Study the drawing (mm; zero at the part's minimum x, y, z) and answer. Give positions to 0.01 mm unless a question says otherwise; leave off trailing zeros. Loops run counter-clockwise (first coordinate to the right, second up) from the corner with the lowest first, then second, coordinate; pieces in that order, holes last. Notation, with made-up numbers: M 66.25,60 L 120.25,60 A19 ccw 120.25,90 Z; hole C 60.5,81 d9. An arc over 180 degrees is marked long. Return JSON: item names as keys, results as strings.
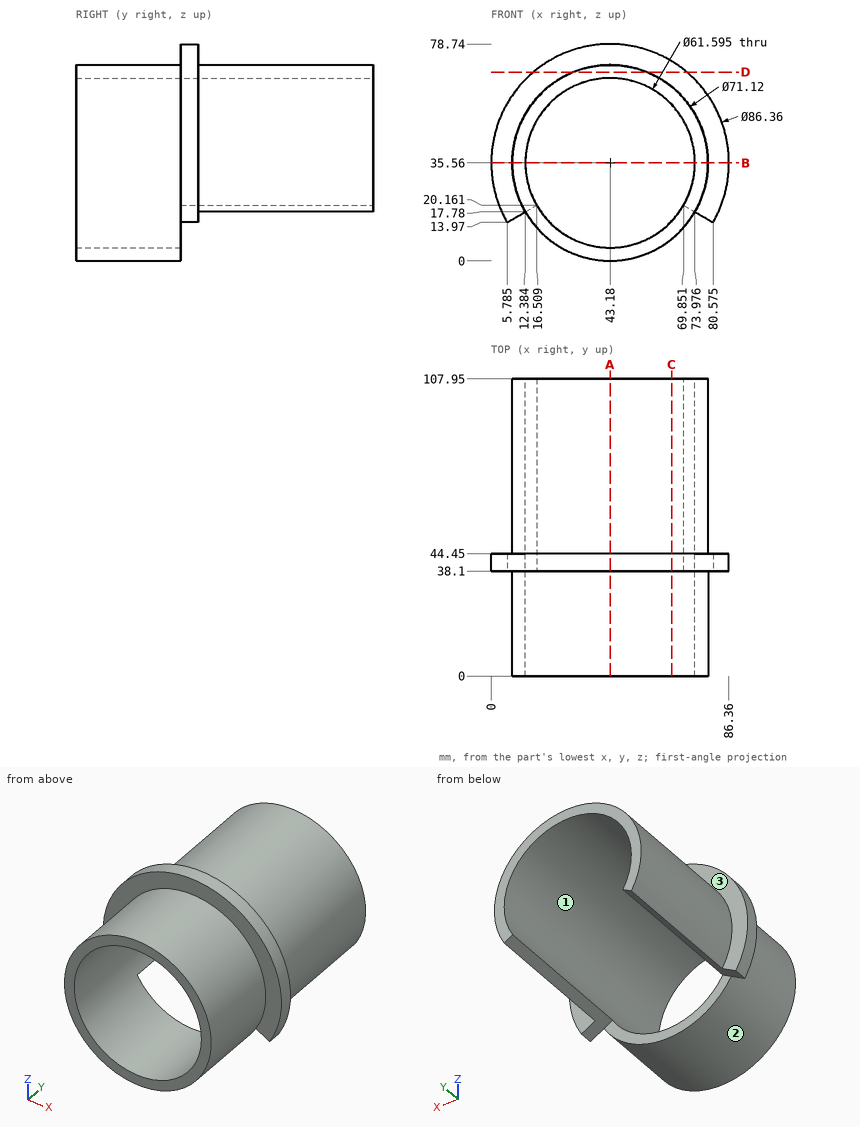
(1) Given pin 1 (1.5 mm diameter, centred on y = 46.5, z = 58.5, fed in from -X); pin 2 (1.5 mm diameter, centred on y = 33.5, z = 28.5, fed in from +X); pin 3 (5 mm diameter, centred on x = 12.5, z = 39, fed in from -Y); pin 4 (4 mm diameter, centred on y = 81.5, z = 47, fed in from -X), each flat-ended and moving along its own axis, determine where each tip first touches the part or whether it passes through.
Values follow:
{"pin 1": "x = 15.39", "pin 2": "x = 78.18", "pin 3": "y = 0", "pin 4": "x = 8.9"}
(2) The part is cut by section A-A (x = 43.18). Determine the outline of the cut face in (y, z).
Values follow:
{"outline": "M 0,0 L 38.1,0 L 38.1,4.76 L 0,4.76 Z; M 0,66.36 L 107.95,66.36 L 107.95,71.12 L 44.45,71.12 L 44.45,78.74 L 38.1,78.74 L 38.1,71.12 L 0,71.12 Z"}
(3) The part is cut by section D-D (z = 68.5). Determine the outline of the cut face in (x, y), and give its area (3 significant figures).
Values follow:
{"outline": "M 15.26,38.1 L 29.78,38.1 L 29.78,0 L 56.58,0 L 56.58,38.1 L 71.1,38.1 L 71.1,44.45 L 56.58,44.45 L 56.58,107.95 L 29.78,107.95 L 29.78,44.45 L 15.26,44.45 Z", "area": "3,080 mm²"}
(4) Straight lines are drawn through the part: line 1 along X through (y, z) = (82.5, 35.56); line 2 along Z through (x, y) = (43.18, 24.5); line 3 along Y through (x, z) = (78, 61). For each, find the intervals that lie inside material, in ascending order.
Values follow:
{"line 1": "7.62 to 12.38, 73.98 to 78.74", "line 2": "0 to 4.76, 66.36 to 71.12", "line 3": "38.1 to 44.45"}
(5) The part is cut by section B-B (z = 35.56). Determine the outline of the cut face in (x, y).
Values follow:
{"outline": "M 0,38.1 L 7.62,38.1 L 7.62,0 L 12.38,0 L 12.38,107.95 L 7.62,107.95 L 7.62,44.45 L 0,44.45 Z; M 73.98,0 L 78.74,0 L 78.74,38.1 L 86.36,38.1 L 86.36,44.45 L 78.74,44.45 L 78.74,107.95 L 73.98,107.95 Z"}
(6) Determine the mould class of the marked faces 1, 2 and 3 for opening direction X: released by +X, released by -X, zero draft, split by the parting line, or undercut.
Values follow:
{"face 1": "undercut", "face 2": "split by the parting line", "face 3": "zero draft"}
(7) The part is cut by section C-C (x = 65.5). Determine the outline of the cut face in (y, z), and give its area (3 significant figures).
Values follow:
{"outline": "M 0,7.88 L 38.1,7.88 L 38.1,14.34 L 0,14.34 Z; M 0,56.78 L 107.95,56.78 L 107.95,63.24 L 44.45,63.24 L 44.45,72.52 L 38.1,72.52 L 38.1,63.24 L 0,63.24 Z", "area": "1,000 mm²"}
